Design review of the part built by this model. Coordinates are the model's own, in mm. A direction names the side the tool comes from. Give positions to 0.01 mm unless a question says otherwise; leave off trailing zeros. Write each loop counter-clockwise with the first axis right and the second up, starting at its lowest first coordinate (ties: lowest second). Pieces come first, ordered by that corner, then holes. Notation, with made-up numbers: (-39.75, -2.75) - (-6.75, -2.75) arc R20 ccw to (-6.75, 7.25) - close; hole circle Ø2 at (82, -11.5). An arc over 180 degrees is marked (long way). Write each question's results on one line, items separated by ' | '. Start each with the question number.
from build123d import *

# Parameters (mm, degrees)
F0_R     = 200
F1_DEPTH = 100
F2_R     = 150
F3_DEPTH = 80
F4_SIZE  = 10
F5_R     = 5
F6_R     = 5


with BuildPart() as f1:
    # F0 (on Top) → F1 (new body)
    with BuildSketch(Plane.XY):
        with Locations((4.4975979886, 0)):
            Circle(F0_R)
    extrude(amount=F1_DEPTH)

    # F2 (on face) → F3 (cut)
    with BuildSketch(Plane.XY.offset(100)):
        Circle(F2_R)
    extrude(amount=-F3_DEPTH, mode=Mode.SUBTRACT)

    # F4
    f4_edges = [f1.edges().sort_by_distance(p)[0] for p in [
        (-195.502402, 0, 100),
    ]]
    chamfer(f4_edges, length=F4_SIZE)

    # F5
    f5_edges = [f1.edges().sort_by_distance(p)[0] for p in [
        (-185.502402, 0, 100),
    ]]
    fillet(f5_edges, radius=F5_R)

    # F6
    f6_edges = [f1.edges().sort_by_distance(p)[0] for p in [
        (-195.502402, 0, 90),
    ]]
    fillet(f6_edges, radius=F6_R)


solid = f1.part
Q1. Add section A-A on z = 27. State the section outline as (x, y) points, plus the area to 3 significant figures.
Q2. Machinability: for faces 4 (the face through (129, -83, 100)), 5 (the face through (-2, 2, 20)), which of the approach directions +Z, -Z, +X, -X, +Y, -Y give a long, thin tool a straight path to every point of the face, cutting with its end or side? Answer none if there is none.
Q3. Insertion check: P1, Ø10, axis at x = -92, z = 24, coming from the -Y side; P2, Ø8, axis at y = -63, z = 18.5, coming from the +X side; P3, Ø3, axis at y = 19, z = 27, coming from the +X side. Each pin has a flat end and moves straight along its axis. Give the tip position at first contact, or say it passes through.
Q4. For line 1 along Y through (x, z) = (0, 49); line 2 along X through (y, z) = (4.5, 87.5); line 3 along Z through (x, y) = (19, 109.5), list the stretches that pass through material, from the lowest coordinate up. Write a range as [from, to].
Q5. The part is to be moulded in two halves that separate along Y. For faces 1 (the face through (-19.527, 148.724, 60.56)), 2 (the face through (-142.91, 135.17, 43.35)), 3 (the face through (2, 3, 0)), say which applies: +Y half, -Y half, draft (parallel to the pull), parting line (faces both ways), or undercut.
Result:
1) outline: circle Ø400 at (4.5, 0); hole circle Ø300 at (0, 0) | area: 55,000 mm²
2) face 4: +Z, +X, -X, +Y, -Y | face 5: +Z
3) P1: stops at y = -177.84 | P2: stops at x = 195.6 | P3: stops at x = 203.73
4) line 1: y = [-199.95, -150], [150, 199.95] | line 2: x = [-195.45, -149.93], [149.93, 204.45] | line 3: z = [0, 20]
5) face 1: undercut | face 2: parting line | face 3: draft
